Answer from the drawing. Dimensions are ordinates in mm from the lowest x, y and z of the part. Round coordinates to 2 decimals unless told otherwise and drop trailing zeros. Order: outer loops, then holes, each group sorted by start corner. A loop starts at its lowest first (then second) coordinate and runs counter-clockwise, first axis right, second up. Notation, with made-up numbers: (29.25, -3) -> (41.25, -3) arc R24 ccw to (41.25, 18) -> close; hole circle Ø1 at (73, 46). An arc over 180 degrees is marked (long way). Use a Markdown table: item, result. Add a question column.
Item 1: Find the intervals of material crossed by L1, parallel to Z at x = 35, y = 0.45; L2, parallel to X at y = 0.85, z = 56; L3, parallel to Z at x = 57, y = 0.7, in increasing order. Write a range as [from, to].
Item 2: A cutting plane is placed at C-C, the plane y = 1.2. Determine the outline of the cut face in (x, z), plus the area to 3 significant figures.
Item 3: A cutting plane is placed at A-A, the plane z = 35. Determine the outline of the cut face in (x, y), plus the area to 3 significant figures.
Item 4: A cutting plane is placed at B-B, the plane x = 35. Determine the outline of the cut face in (y, z), plus the area to 3 significant figures.
Item 5: A cutting plane is placed at D-D, the plane z = 57. Determine the outline of the cut face in (x, y).
Item 6: Flat-ended cylindrical pins translate along their axes: P1, Ø0.5, axis at x = 33.5, y = 1, coming from the +Z side; P2, Ø2.5, axis at x = 13, z = 13, coming from the -Y side; P3, Ø0.8, axis at y = 1, z = 40, coming from the -X side; P4, Ø0.5, axis at x = 34.5, y = 1, coming from the -Z side. Find the tip coordinate at first contact, or state that the pin passes through.
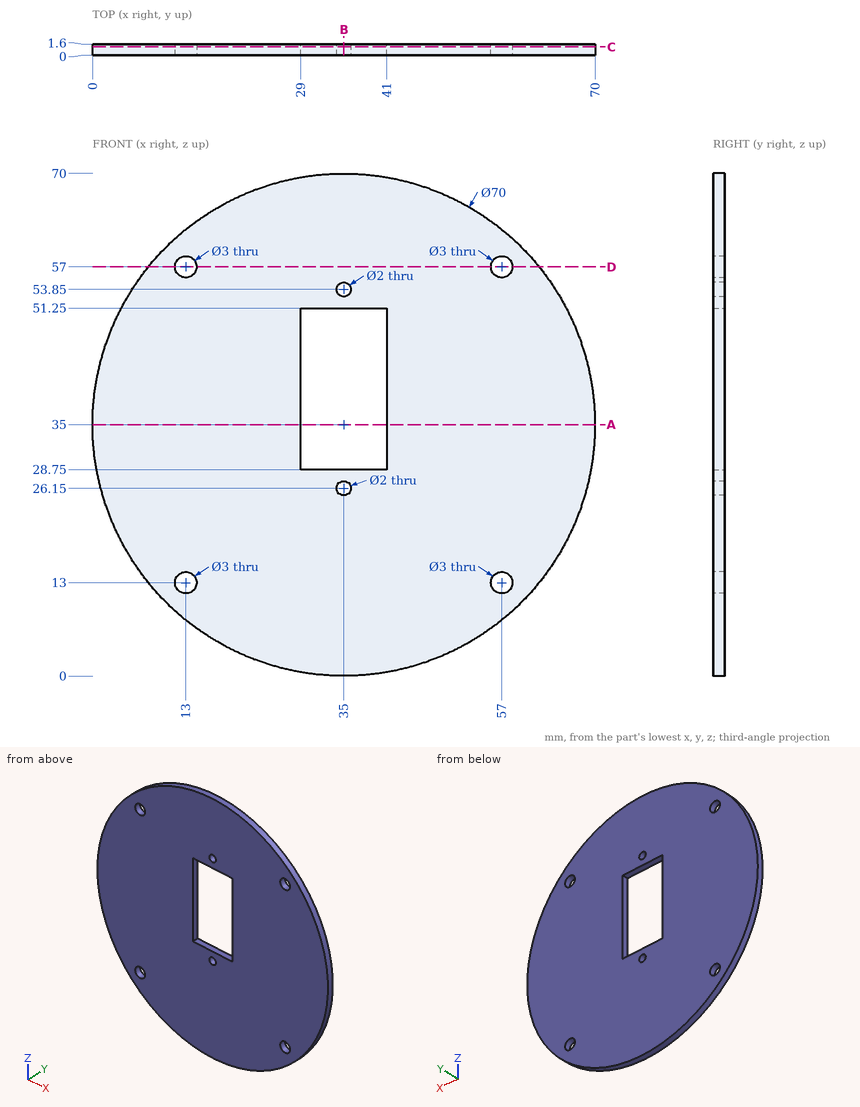
Reported:
| question | item | result |
|---|---|---|
| 1 | L1 | [0, 25.15], [27.15, 28.75], [51.25, 52.85], [54.85, 70] |
| 1 | L2 | [7, 11.88], [14.12, 55.88], [58.12, 63] |
| 1 | L3 | [7.78, 11.5], [14.5, 55.5], [58.5, 62.22] |
| 2 | outline | circle Ø70 at (35, 35); hole circle Ø3 at (13, 13); hole circle Ø3 at (13, 57); hole (29, 28.75) -> (41, 28.75) -> (41, 51.25) -> (29, 51.25) -> close; hole circle Ø2 at (35, 26.15); hole circle Ø2 at (35, 53.85); hole circle Ø3 at (57, 13); hole circle Ø3 at (57, 57) |
| 2 | area | 3,540 mm² |
| 3 | outline | (0, 0) -> (29, 0) -> (29, 1.6) -> (0, 1.6) -> close; (41, 0) -> (70, 0) -> (70, 1.6) -> (41, 1.6) -> close |
| 3 | area | 92.8 mm² |
| 4 | outline | (0, 0) -> (1.6, 0) -> (1.6, 25.15) -> (0, 25.15) -> close; (0, 27.15) -> (1.6, 27.15) -> (1.6, 28.75) -> (0, 28.75) -> close; (0, 51.25) -> (1.6, 51.25) -> (1.6, 52.85) -> (0, 52.85) -> close; (0, 54.85) -> (1.6, 54.85) -> (1.6, 70) -> (0, 70) -> close |
| 4 | area | 69.6 mm² |
| 5 | outline | (7.78, 0) -> (11.5, 0) -> (11.5, 1.6) -> (7.78, 1.6) -> close; (14.5, 0) -> (55.5, 0) -> (55.5, 1.6) -> (14.5, 1.6) -> close; (58.5, 0) -> (62.22, 0) -> (62.22, 1.6) -> (58.5, 1.6) -> close |
| 6 | P1 | z = 69.98 |
| 6 | P2 | through |
| 6 | P3 | x = 0.3 |
| 6 | P4 | z = 0 |
